For this review, take the finished solid that the model builds, in its own axes (mm). Round coordinates to 2 decimals unless told otherwise and drop trailing zeros. Write each loop counter-clockwise with the first axis right and the second up, starting at its lowest first coordinate (ties: lowest second). Pieces come first, ordered by that corner, then holes. Notation, with made-up numbers: M -21.75,62.25 L -12.75,62.25 A16 ccw -12.75,72.25 Z; hole C 13,56.5 d9. An arc over 180 degrees is marked long. Use one line per item in the form item = value. Start each with the question number.
Item 1: Add section A-A (x = 21). State the section outline as (y, z) points, and give its area (3 significant figures).
Item 2: Add section C-C (x = 31). State the section outline as (y, z) points.
Item 3: For line 1 (Y direction, x = 11, z = 8.5); line 2 (Y direction, x = 21, z = 6.5), list the stretches that pass through material, from the lowest coordinate up. Write a range as [from, to].
Item 4: Add section B-B (y = -82). State the section outline as (x, z) points, and give its area (3 significant figures).
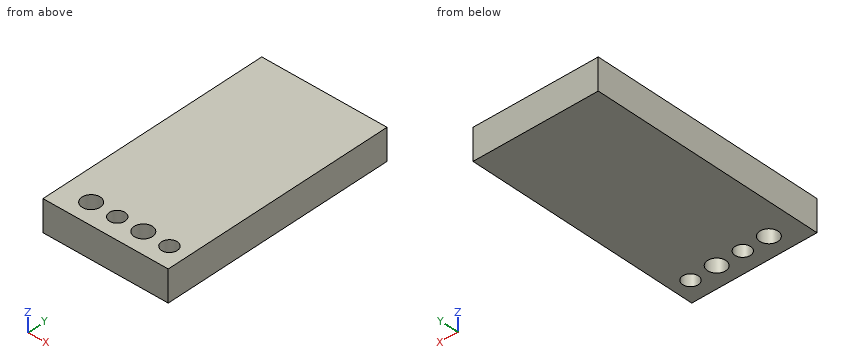
from build123d import *

# Parameters (mm, degrees)
F0_W     = 48
F0_H     = 90
F1_DEPTH = 12
F3_D     = 7
F3_DEPTH = 12
F4_D     = 6
F4_DEPTH = 12


with BuildPart() as f1:
    # F0 (on Top) → F1 (new body)
    with BuildSketch(Plane.XY):
        with Locations((24, -45)):
            Rectangle(F0_W, F0_H)
    extrude(amount=F1_DEPTH)

    # F3
    with Locations(Plane.XY.offset(12)):
        with Locations((11, -82), (31, -82)):
            Hole(F3_D / 2, depth=F3_DEPTH)

    # F4
    with Locations(Plane.XY.offset(12)):
        with Locations((21, -82), (41, -82)):
            Hole(F4_D / 2, depth=F4_DEPTH)


solid = f1.part
Calculated:
q1.outline = M -90,0 L -85,0 L -85,12 L -90,12 Z; M -79,0 L 0,0 L 0,12 L -79,12 Z
q1.area = 1,010 mm^2
q2.outline = M -90,0 L -85.5,0 L -85.5,12 L -90,12 Z; M -78.5,0 L 0,0 L 0,12 L -78.5,12 Z
q3.line_1 = [-90, -85.5], [-78.5, 0]
q3.line_2 = [-90, -85], [-79, 0]
q4.outline = M 0,0 L 7.5,0 L 7.5,12 L 0,12 Z; M 14.5,0 L 18,0 L 18,12 L 14.5,12 Z; M 24,0 L 27.5,0 L 27.5,12 L 24,12 Z; M 34.5,0 L 38,0 L 38,12 L 34.5,12 Z; M 44,0 L 48,0 L 48,12 L 44,12 Z
q4.area = 264 mm^2
